from build123d import *

# Parameters (mm, degrees)
F0_R     = 6.2011167501
F0_R_2   = 4.0462607589
F1_DEPTH = 12.7


with BuildPart() as f1:
    # F0 (on Front) → F1 (new body, symmetric)
    with BuildSketch(Plane.XZ):
        with BuildLine():
            Line((35.7664418355, 15.0339733809), (-46.7835581645, 15.0339733809))
            Line((-46.7835581645, 15.0339733809), (-46.7835581645, -15.0339733809))
            Line((-46.7835581645, -15.0339733809), (35.7664418355, -15.0339733809))
            ThreePointArc((35.7664418355, -15.0339733809), (40.256569896, -13.1741014415), (42.1164418355, -8.6839733809))
            Line((42.1164418355, -8.6839733809), (42.1164418355, 8.6839733809))
            ThreePointArc((42.1164418355, 8.6839733809), (40.256569896, 13.1741014415), (35.7664418355, 15.0339733809))
        make_face()
        with Locations((-27.7343895286, 0)):
            Circle(F0_R, mode=Mode.SUBTRACT)
        with Locations((14.892292209, 0)):
            Circle(F0_R_2, mode=Mode.SUBTRACT)
    extrude(amount=F1_DEPTH, both=True)


solid = f1.part
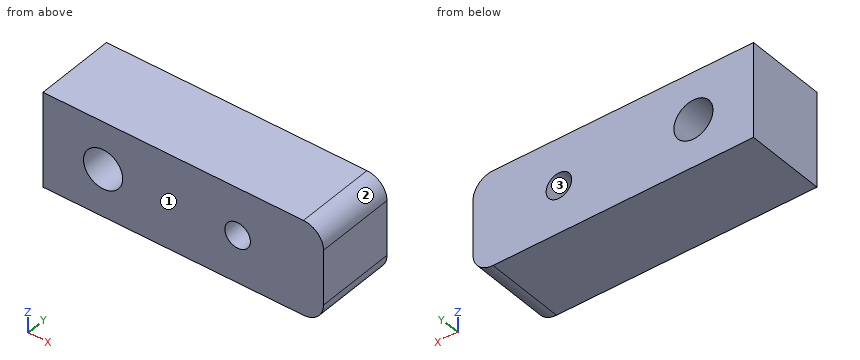
Input: part model. Units: mm. Frame: model coordinates. Face numbers are marked on the shaded views. Give positions to 0.01 mm unless a question says otherwise; leave off trailing zeros. Order: outer loops, then holes, each group sorted by start corner. A loop starts at its lowest first (then second) coordinate and runs counter-clockwise, first axis right, second up. Notation, with made-up numbers: (75, -39) -> (96, -39) arc R17 cw to (96, -7) -> close; hole circle Ø6 at (53, -39). An arc over 180 degrees is marked (long way). Use one line per item in the form item = value.
1) First-contact query: pin 1 Ø10 at (x, z) = (-27.73, 0) entering from +Y. Flat tip, straight axial feed; report the tip coordinate or a pass-through.
Response values:
pin_1 = through
2) Section A-A, the plane z = 0. Return loops of the section in (x, y).
Response values:
outline = (-46.78, -12.7) -> (-33.94, -12.7) -> (-33.94, 12.7) -> (-46.78, 12.7) -> close; (-21.53, -12.7) -> (10.85, -12.7) -> (10.85, 12.7) -> (-21.53, 12.7) -> close; (18.94, -12.7) -> (42.12, -12.7) -> (42.12, 12.7) -> (18.94, 12.7) -> close
3) Section C-C, the plane x = -27.5. Return loops of the section in (y, z).
Response values:
outline = (-12.7, -15.03) -> (12.7, -15.03) -> (12.7, -6.2) -> (-12.7, -6.2) -> close; (-12.7, 6.2) -> (12.7, 6.2) -> (12.7, 15.03) -> (-12.7, 15.03) -> close
4) Line query: probe 1 along Z at (x, y) = (-27.5, 5.5); probe 2 along X at (y, z) = (-5.75, 0.5); probe 3 along X at (y, z) = (11.75, 3.5). Output: solid intervals per line, ascending.
Response values:
probe_1 = -15.03 to -6.2, 6.2 to 15.03
probe_2 = -46.78 to -33.92, -21.55 to 10.88, 18.91 to 42.12
probe_3 = -46.78 to -32.85, -22.62 to 12.86, 16.92 to 42.12
5) Mould query, pull axis X, two halves, no side actions, for the marked faces 1, 2 and 3. Classes: pulls with the +X half, pulls with the -X half, needs draft (parallel to the pull), parting line crosses it, or undercut.
Response values:
face_1 = needs draft
face_2 = pulls with the +X half
face_3 = undercut
6) Section D-D, the plane z = 5. Return loops of the section in (x, y).
Response values:
outline = (-46.78, -12.7) -> (-31.4, -12.7) -> (-31.4, 12.7) -> (-46.78, 12.7) -> close; (-24.07, -12.7) -> (42.12, -12.7) -> (42.12, 12.7) -> (-24.07, 12.7) -> close
7) Section B-B, the plane y = -1.75. Return loops of the section in (x, z).
Response values:
outline = (-46.78, -15.03) -> (35.77, -15.03) arc R6.35 ccw to (42.12, -8.68) -> (42.12, 8.68) arc R6.35 ccw to (35.77, 15.03) -> (-46.78, 15.03) -> close; hole circle Ø12.4 at (-27.73, 0); hole circle Ø8.09 at (14.89, 0)
